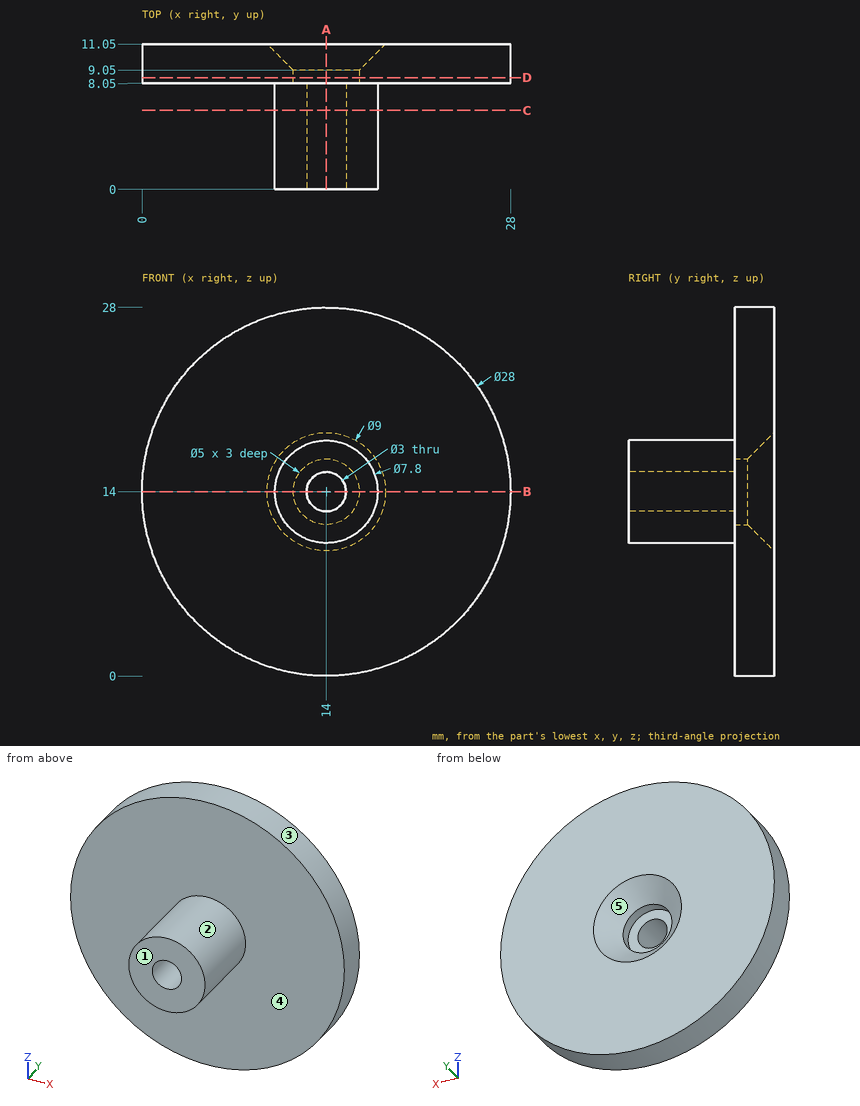
Job drawing, mm, ordinate dimensions from the low corner. One solid piece. A direction names the side the tool comes from. Give positions to 0.01 mm unless a question says otherwise; leave off trailing zeros. Write each loop counter-clockwise with the first axis right and the second up, starting at its lowest first coordinate (ties: lowest second). Pieces come first, ordered by that corner, then holes. Notation, with made-up numbers: M 48,36 L 67,36 A26 ccw 67,51 Z; hole C 18.5,32.5 d1. An arc over 180 degrees is marked long. One line per item, written item: value. Start each with the question number.
Q1. Saw through at A-A, the plane x = 14. Write the cut outline in (y, z).
Q2. Two-plate mould, pull along Z, no slides. Class the marked faces 3, 4 and 5: +Z half, -Z half, draft (parallel to the pull), parting line (faces both ways), or undercut.
Q3. Drop flat-ended pins along their axis: pin 1 Ø4 at (x, z) = (24, 15) entering from -Y; pin 2 Ø8 at (x, z) = (14, 14) entering from +Y; pin 3 Ø3.5 at (x, z) = (14, 14) entering from -Y; pin 4 Ø1.5 at (y, z) = (8.5, 10.5) entering from +X. Give the stop position or say it passes through.
Q4. Probe probe 1 along Z at (x, y) = (14, 8.55); probe 2 along Y at (x, z) = (3.5, 13.25). List the from-to ranges inside material, lowest first. Write a range as [from, to].
Q5. Saw through at D-D, the plane y = 8.5. Write the cut outline in (x, z), plus the area to 3 significant figures.
Q6. 3-axis set-ups, long thin cutter, end or side, ignore diameter. For the marked faces 1 and 2: which of +Z, -Z, +X, -X, +Y, -Y reach the whole face in a straight line?
Q7. Saw through at C-C, the plane y = 6. Write the cut outline in (x, z), plus the area to 3 significant figures.
Q8. Saw through at B-B, the plane z = 14. Write the cut outline in (x, y).
Output values:
1. outline: M 0,10.1 L 8.05,10.1 L 8.05,0 L 11.05,0 L 11.05,9.5 L 9.05,11.5 L 8.05,11.5 L 8.05,12.5 L 0,12.5 Z; M 0,15.5 L 8.05,15.5 L 8.05,16.5 L 9.05,16.5 L 11.05,18.5 L 11.05,28 L 8.05,28 L 8.05,17.9 L 0,17.9 Z
2. face 3: parting line
2. face 4: draft
2. face 5: undercut
3. pin 1: stops at y = 8.05
3. pin 2: stops at y = 10.55
3. pin 3: stops at y = 0
3. pin 4: stops at x = 27.73
4. probe 1: z = [0, 11.5], [16.5, 28]
4. probe 2: y = [8.05, 11.05]
5. outline: C 14,14 d28; hole C 14,14 d5
5. area: 596 mm²
6. face 1: +Z, -Z, +X, -X, -Y
6. face 2: -Y
7. outline: C 14,14 d7.8; hole C 14,14 d3
7. area: 40.7 mm²
8. outline: M 0,8.05 L 10.1,8.05 L 10.1,0 L 12.5,0 L 12.5,8.05 L 11.5,8.05 L 11.5,9.05 L 9.5,11.05 L 0,11.05 Z; M 15.5,0 L 17.9,0 L 17.9,8.05 L 28,8.05 L 28,11.05 L 18.5,11.05 L 16.5,9.05 L 16.5,8.05 L 15.5,8.05 Z
